from build123d import *

# Parameters (mm, degrees)
SKETCH1_W          = 130
SKETCH1_H          = 69
BASE_FLANGE1_DEPTH = 10
SKETCH6_R          = 10
SKETCH6_R_2        = 6
CUT_EXTRUDE1_DEPTH = 75.264729179
FILLET1_R          = 10
CUT_EXTRUDE2_DEPTH = 75.264729179
FILLET2_R          = 3


# Sheet-metal steps are written as plain solids
with BuildPart() as part:
    # Sketch1 → Base-Flange1 (new body)
    with BuildSketch(Plane.XY):
        Rectangle(SKETCH1_W, SKETCH1_H)
    extrude(amount=-BASE_FLANGE1_DEPTH)

    # Sketch6 → Cut-Extrude1 (cut, through all)
    with BuildSketch(Plane.XY):
        Circle(SKETCH6_R)
        with Locations((-40, 20)):
            Circle(SKETCH6_R_2)
        with Locations((-40, -20)):
            Circle(SKETCH6_R_2)
        with Locations((40, -20)):
            Circle(SKETCH6_R_2)
        with Locations((40, 20)):
            Circle(SKETCH6_R_2)
    extrude(amount=-CUT_EXTRUDE1_DEPTH, mode=Mode.SUBTRACT)

    # Fillet1
    fillet1_edges = [part.edges().sort_by_distance(p)[0] for p in [
        (-65, 34.5, -5),
        (65, 34.5, -5),
    ]]
    fillet(fillet1_edges, radius=FILLET1_R)

    # Sketch7 → Cut-Extrude2 (cut, through all)
    with BuildSketch(Plane.XY):
        with BuildLine():
            Line((67, 34.5), (67, 30.5))
            ThreePointArc((67, 30.5), (61, 24.5), (55, 30.5))
            Line((55, 30.5), (55, 34.5))
            ThreePointArc((55, 34.5), (61, 40.5), (67, 34.5))
        make_face()
    extrude(amount=-CUT_EXTRUDE2_DEPTH, mode=Mode.SUBTRACT)

    # Fillet2
    fillet2_edges = [part.edges().sort_by_distance(p)[0] for p in [
        (55, 34.5, -5),
        (64.896192513, 25.93714082, -5),
    ]]
    fillet(fillet2_edges, radius=FILLET2_R)


solid = part.part
Build history of the part. All positions in model axes, mm. Round coordinates to 2 decimals unless told otherwise and drop trailing zeros. Write each loop counter-clockwise with the first axis right and the second up, starting at its lowest first coordinate (ties: lowest second). Pieces come first, ordered by that corner, then holes. Notation, with made-up numbers: (54.5, 38) -> (79.5, 38) arc R21 cw to (79.5, 52) -> close; hole circle Ø5 at (-23.5, -39). An arc over 180 degrees is marked (long way). Use one line per item in the form item = value.
Q1. Drill centre lines: L1, parallel to Y at x = -40, z = -5.75; L2, parallel to X at y = -19.5, z = -6.75; L3, parallel to Y at x = -41, z = -9. Where is each one in solid material? Low to high.
Conclusion:
L1 = -34.5 to -26, -14 to 14, 26 to 34.5
L2 = -65 to -45.98, -34.02 to 34.02, 45.98 to 65
L3 = -34.5 to -25.92, -14.08 to 14.08, 25.92 to 34.5
Q2. Two-plate mould, pull along X, no slides. Class faces 1 (the cylindrical face through (-2.17, -9.76, -4.93)), 2 (the flat face through (65, -7, -5)), 3 (the cylindrical face through (34, 20, -5)), 4 (the flat face through (-2, 34.5, -5)): released by +X, released by -X, zero draft, split by the parting line, or undercut.
Conclusion:
face_1 = undercut
face_2 = released by +X
face_3 = undercut
face_4 = zero draft
Q3. Band-saw the part on D-D, the plane x = 0. Write the cut outline in (y, z), then the cut area to 3 significant figures.
Conclusion:
outline = (-34.5, -10) -> (-10, -10) -> (-10, 0) -> (-34.5, 0) -> close; (10, -10) -> (34.5, -10) -> (34.5, 0) -> (10, 0) -> close
area = 490 mm²
Q4. Band-saw the part on C-C, the plane x = 40. Write the cut outline in (y, z), then the cut area to 3 significant figures.
Conclusion:
outline = (-34.5, -10) -> (-26, -10) -> (-26, 0) -> (-34.5, 0) -> close; (-14, -10) -> (14, -10) -> (14, 0) -> (-14, 0) -> close; (26, -10) -> (34.5, -10) -> (34.5, 0) -> (26, 0) -> close
area = 450 mm²
Q5. Drop a flat-ended pin along its axis: P1, Ø0.8, axis at y = 31, z = -5, coming from the +X side. Give the stop position or say it passes through.
Conclusion:
P1 = 55
Q6. Band-saw the part on A-A, the plane y = -20. Write the cut outline in (x, z).
Conclusion:
outline = (-65, -10) -> (-46, -10) -> (-46, 0) -> (-65, 0) -> close; (-34, -10) -> (34, -10) -> (34, 0) -> (-34, 0) -> close; (46, -10) -> (65, -10) -> (65, 0) -> (46, 0) -> close
Q7. Band-saw the part on B-B, the plane y = 0. Write the cut outline in (x, z).
Conclusion:
outline = (-65, -10) -> (-10, -10) -> (-10, 0) -> (-65, 0) -> close; (10, -10) -> (65, -10) -> (65, 0) -> (10, 0) -> close
